Build history of the part. All positions in model axes, mm. Face numbers are marked on the shaded views. Round coordinates to 2 decimals unless told otherwise and drop trailing zeros. Loops run counter-clockwise (first coordinate to the right, second up) from the corner with the lowest first, then second, coordinate; pieces in that order, holes last.
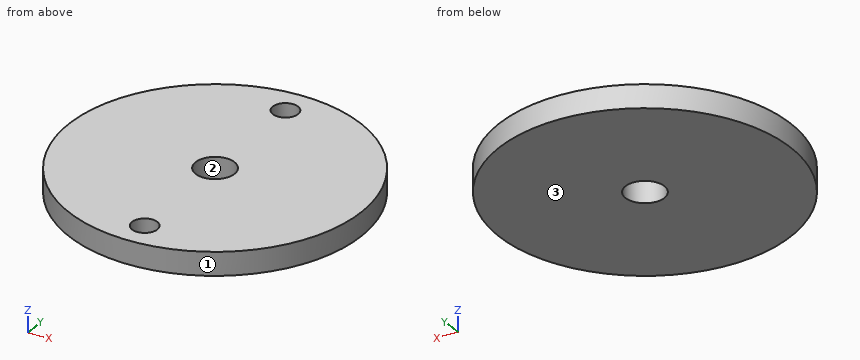
Autodesk Inventor part; units mm, degrees
ref_plane "YZ Plane" through (0, 0, 0) normal (1, 0, 0) x (0, 1, 0)
ref_plane "XZ Plane" through (0, 0, 0) normal (0, 1, 0) x (-1, 0, 0)
ref_plane "XY Plane" through (0, 0, 0) normal (0, 0, 1) x (1, 0, 0)
sketch "草圖1" plane through (0, 0, 0) normal (0, 0, 1) x (1, 0, 0)
  circle A0 centre (0, 0) radius 75
  dimension "d0" = 150
extrude "擠出1" add sketch "草圖1" along normal blind 12
sketch "草圖2" plane through (0, 0, 12) normal (0, 0, 1) x (1, 0, 0)
  circle A0 centre (0, 0) radius 75
  line L0 (0, 0) -> (0, -60)
  circle A1 centre (0, -60) radius 6.5
  dimension "d3" = 60
  dimension "d4" = 13
extrude "擠出2" cut sketch "草圖2" against normal blind 11 contours A1
fillet "圓角1" radius 4 1 edges at (-6.5, -60, 1)
pattern_circular "環形陣列1" count 2 over 360 about axis through (0, 0, 0) along (0, 0, 1) of "擠出2", "圓角1"
sketch "草圖3" plane through (0, 0, 12) normal (0, 0, 1) x (1, 0, 0)
  circle A0 centre (0, 0) radius 75
  circle A1 centre (0, 0) radius 10
  dimension "d11" = 20
extrude "擠出3" cut sketch "草圖3" against normal blind 12 contours A1
(1) Pull direction X, two halves, no side cores. Call the marked faces 1, 2 and 3: +X half, -X half, draft (parallel to the pull), parting line (faces both ways), or undercut.
Responses:
face 1: parting line
face 2: undercut
face 3: draft
(2) Slice it at A-A on y = 0. List the corners of the cut face in (x, z).
Responses:
outline: (-75, 0) - (-10, 0) - (-10, 12) - (-75, 12) - close; (10, 0) - (75, 0) - (75, 12) - (10, 12) - close
(3) Pin check, flat tips, straight feed: P1, Ø10.5, axis at x = 0, y = 60, coming from the -Z side; P2, Ø1.5, axis at y = -59, z = 8, coming from the +X side; P3, Ø8, axis at x = 0, y = -60, coming from the +Z side; P4, Ø5.5, axis at x = 1, y = -60.5, coming from the +Z side. Stop position of each tip, or through.
Responses:
P1: stops at z = 0
P2: stops at x = 47.24
P3: stops at z = 1.29
P4: stops at z = 1.24
(4) Slice it at C-C on y = -32.5. List the corners of the cut face in (x, z).
Responses:
outline: (-67.59, 0) - (67.59, 0) - (67.59, 12) - (-67.59, 12) - close
(5) Probe line 1 (Y direction, x = 0, z = 9.25); line 2 (Y direction, x = 4, z = 3.5); line 3 (X direction, y = 5.5, z = 3). List the from-to ranges inside material, lowest first.
Responses:
line 1: y = -75 to -66.5, -53.5 to -10, 10 to 53.5, 66.5 to 75
line 2: y = -74.89 to -64.75, -55.25 to -9.17, 9.17 to 55.25, 64.75 to 74.89
line 3: x = -74.8 to -8.35, 8.35 to 74.8
(6) Slice it at D-D on z = 3. Count the separate pieces of the cut face and the enclosed holes in it, plus the area to 3 significant figures.
Responses:
separate pieces: 1
enclosed holes: 3
area: 17,100 mm2
(7) Slice it at B-B on x = -60. List the corners of the cut face in (y, z), plus the area to 3 significant figures.
Responses:
outline: (-45, 0) - (45, 0) - (45, 12) - (-45, 12) - close
area: 1,080 mm2
